CAD build for the part. Positions are in the model's coordinates, mm. Face numbers are marked on the shaded views. A direction names the side the tool comes from. Round coordinates to 2 decimals unless told otherwise and drop trailing zeros. Loops run counter-clockwise (first coordinate to the right, second up) from the corner with the lowest first, then second, coordinate; pieces in that order, holes last. Notation, with made-up numbers: (49, 60) - (75, 60) arc R14 cw to (75, 71) - close; hole circle Ø7 at (77, -20). An arc over 180 degrees is marked (long way). Use one line per item in the form item = value.
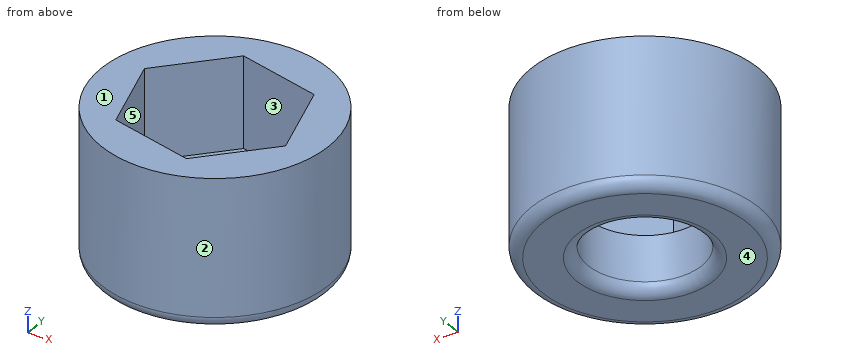
from build123d import *

# Parameters (mm, degrees)
F0_R     = 10
F0_R_2   = 5
F1_DEPTH = 5
F2_DEPTH = 8
F3_R     = 1


with BuildPart() as f1:
    # F0 (on Top) → F1 (new body)
    with BuildSketch(Plane.XY):
        Circle(F0_R)
        Polygon((-7.325631, 1.633545), (-2.248124, 7.160955), (5.077507, 5.52741), (7.325631, -1.633545), (2.248124, -7.160955), (-5.077507, -5.52741), align=None, mode=Mode.SUBTRACT)
        Polygon((5.077507, 5.52741), (-2.248124, 7.160955), (-7.325631, 1.633545), (-5.077507, -5.52741), (2.248124, -7.160955), (7.325631, -1.633545), align=None)
        Circle(F0_R_2, mode=Mode.SUBTRACT)
    extrude(amount=-F1_DEPTH)

    # F0 (on Top) → F2 (join)
    with BuildSketch(Plane.XY):
        Circle(F0_R)
        Polygon((-7.325631, 1.633545), (-2.248124, 7.160955), (5.077507, 5.52741), (7.325631, -1.633545), (2.248124, -7.160955), (-5.077507, -5.52741), align=None, mode=Mode.SUBTRACT)
    extrude(amount=F2_DEPTH)

    # F3
    f3_edges = [f1.edges().sort_by_distance(p)[0] for p in [
        (-10, 0, -5),
        (-5, 0, -5),
    ]]
    fillet(f3_edges, radius=F3_R)


solid = f1.part
1) Two-plate mould, pull along Y, no slides. Class the marked faces 1, 2 and 3: +Y half, -Y half, draft (parallel to the pull), parting line (faces both ways), or undercut.
Report:
face_1 = draft
face_2 = parting line
face_3 = undercut
2) Slice it at C-C (x = 0). Write the cut outline in (y, z), plus the area to 3 significant figures.
Report:
outline = (-10, -4) arc R1 ccw to (-9, -5) - (-6, -5) arc R1 ccw to (-5, -4) - (-5, 0) - (-6.66, 0) - (-6.66, 8) - (-10, 8) - close; (5, -4) arc R1 ccw to (6, -5) - (9, -5) arc R1 ccw to (10, -4) - (10, 8) - (6.66, 8) - (6.66, 0) - (5, 0) - close
area = 103 mm^2
3) Tool access for the marked faces 4 and 5: list every direction of +Z, -Z, +X, -X, +Y, -Y with a clear straight run to the whole face (end or side of a thin tool).
Report:
face_4 = -Z, +X, -X, +Y, -Y
face_5 = +Z
4) Drill centre lines: probe 1 along Y at (x, z) = (0, -0.9); probe 2 along Y at (x, z) = (-8, 2.75); probe 3 along X at (y, z) = (4.5, 1.5). Where is each one in solid material? Low to high.
Report:
probe_1 = -10 to -5, 5 to 10
probe_2 = -6 to 6
probe_3 = -8.93 to -4.69, 5.4 to 8.93
5) Slice it at B-B (y = 0). Write the cut outline in (x, z).
Report:
outline = (-10, -4) arc R1 ccw to (-9, -5) - (-6, -5) arc R1 ccw to (-5, -4) - (-5, 0) - (-6.81, 0) - (-6.81, 8) - (-10, 8) - close; (5, -4) arc R1 ccw to (6, -5) - (9, -5) arc R1 ccw to (10, -4) - (10, 8) - (6.81, 8) - (6.81, 0) - (5, 0) - close
6) Flat gauge pins, fed straight in: pin 1 (1 mm diameter, centred on y = -5, z = 2, fed in from -X); pin 2 (3 mm diameter, centred on x = -4, z = 1.5, fed in from +Y); pin 3 (3 mm diameter, centred on y = 4, z = 2, fed in from -X); pin 4 (8 mm diameter, centred on x = 0, y = 0, fed in from +Z). Where does each tip first touch, or does it go through?
Report:
pin_1 = -8.93
pin_2 = 9.68
pin_3 = -9.68
pin_4 = through
7) Slice it at A-A (z = 6.5). Write the cut outline in (x, y), plus the area to 3 significant figures.
Report:
outline = circle Ø20 at (0, 0); hole (-7.33, 1.63) - (-5.08, -5.53) - (2.25, -7.16) - (7.33, -1.63) - (5.08, 5.53) - (-2.25, 7.16) - close
area = 168 mm^2
